Design review of the part shown in the three views and the two pictorial views. Dimensions are in mm from the part's minimum x, y and z. A direction names the side the tool comes from. Coordinates: 2 decimals unless noted, no trailing zeros. Write each loop counter-clockwise with the first axis right and the second up, starting at its lowest first coordinate (ties: lowest second). Pieces come first, ordered by that corner, then holes. Notation, with made-up numbers: (81.5, 36) - (108.5, 36) arc R26 cw to (108.5, 50) - close; hole circle Ø5 at (-15.75, 11). An arc over 180 degrees is marked (long way). Return JSON: item names as keys, results as strings. Group by question number.
(1) Tool access review of the marked faces 1, 2 and 3: name each direction out of +Z, -Z, +X, -X, +Y, -Y from which nothing blocks a thin tool from reaching the whole face with its end or side.
(2) To check wall thickness, follow L1, parallel to Y at x = 1.85, z = 2.05; L2, parallel to Y at x = 3.55, z = 4.5; L3, parallel to X at y = 10, z = 3.7. State the ranges of each line that lie inside material, in increasing order. Write a range as from..to.
(3) We need section A-A on x = 2.5. State the section outline as (y, z) points, then the cut area to 3 significant figures.
(4) For pin 1 Ø3 at (y, z) = (11, 1.5) entering from +X; pin 2 Ø1.9 at (x, z) = (3, 2.5) entering from +Y; pin 3 Ø1.5 at (y, z) = (7.5, 1) entering from -X; pin 4 Ø2 at (y, z) = (6, 2.5) entering from -X, all flat-tipped, find the tip position at first contact; note any pin that passes through.
(5) Draft analysis for pull direction Z (two halves, no side actions). For the marked faces 4, 5 and 6, state which applies: released by +Z, released by -Z, zero draft, split by the parting line, or undercut.
(6) We need section B-B on y = 7.75. State the section outline as (x, z) points, then the cut area to 3 significant figures.
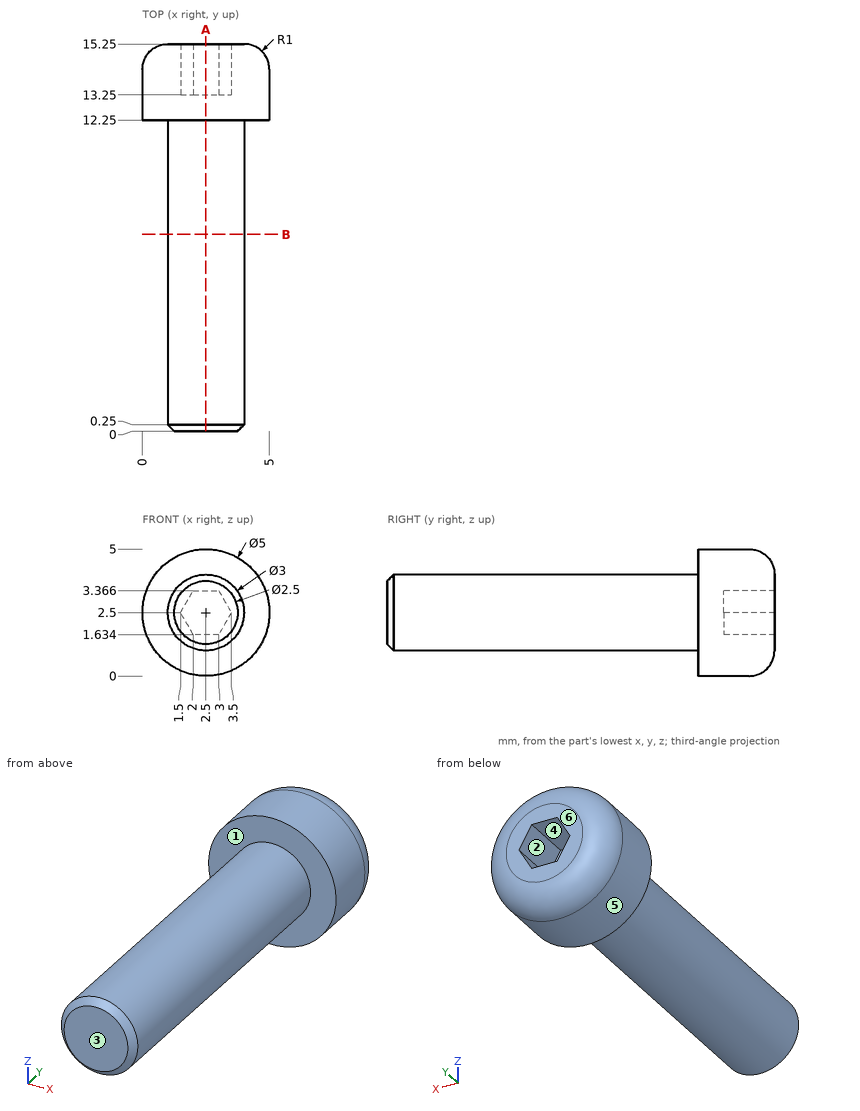
Ans:
{
 "1": {"face 1": "-Y", "face 2": "+Y", "face 3": "+Z, -Z, +X, -X, -Y"},
 "2": {"L1": "0..13.25", "L2": "12.25..14.9", "L3": "1.6..3.4"},
 "3": {"outline": "(0, 1.25) - (0.25, 1) - (12.25, 1) - (12.25, 0) - (14.25, 0) arc R1 ccw to (15.25, 1) - (15.25, 1.63) - (13.25, 1.63) - (13.25, 3.37) - (15.25, 3.37) - (15.25, 4) arc R1 ccw to (14.25, 5) - (12.25, 5) - (12.25, 4) - (0.25, 4) - (0, 3.75) - close", "area": "47.8 mm²"},
 "4": {"pin 1": "x = 4.99", "pin 2": "y = 15.25", "pin 3": "x = 1.2", "pin 4": "x = 1"},
 "5": {"face 4": "undercut", "face 5": "split by the parting line", "face 6": "zero draft"},
 "6": {"outline": "circle Ø3 at (2.5, 2.5)", "area": "7.07 mm²"}
}
